from build123d import *

# Parameters (mm, degrees)
F0_W     = 10
F0_H     = 12
F0_W_2   = 7.6
F0_H_2   = 10
F1_DEPTH = 0.75
F0_W_3   = 6.8
F0_H_3   = 9.2
F2_DEPTH = 1.5
F3_R     = 1


with BuildPart() as f1:
    # F0 (on Top) → F1 (new body)
    with BuildSketch(Plane.XY):
        Rectangle(F0_W, F0_H)
        Rectangle(F0_W_2, F0_H_2, mode=Mode.SUBTRACT)
    extrude(amount=F1_DEPTH)

    # F0 (on Top) → F2 (join)
    with BuildSketch(Plane.XY):
        Rectangle(F0_W_2, F0_H_2)
        Rectangle(F0_W_3, F0_H_3, mode=Mode.SUBTRACT)
    extrude(amount=F2_DEPTH)

    # F3
    f3_edges = [f1.edges().sort_by_distance(p)[0] for p in [
        (5, 6, 0.375),
        (-5, 6, 0.375),
        (-5, -6, 0.375),
        (5, -6, 0.375),
    ]]
    fillet(f3_edges, radius=F3_R)


solid = f1.part
Work out the finished part from the listing and answer in its coordinate system (mm). A direction names the side the tool comes from. Give positions to 0.01 mm unless a question says otherwise; leave off trailing zeros. Order: outer loops, then holes, each group sorted by start corner. A loop starts at its lowest first (then second) coordinate and runs counter-clockwise, first axis right, second up. Notation, with made-up numbers: (-3.5, 79.5) -> (44.5, 79.5) arc R20 ccw to (44.5, 116.5) -> close; hole circle Ø11 at (-32, -3.5). An arc over 180 degrees is marked (long way). One line per item, written item: value.
Item 1: A tool of negligible diameter and unlimited length cuts with its end or side. For faces 1 (the cylindrical face through (-4.715, 5.699, 0.38)), 2 (the flat face through (0, 4.6, 1)), from which of +Z, -Z, +X, -X, +Y, -Y can it reach the whole face along a straight path? Write none if from no direction.
Answer sheet:
face 1: +Z, -Z, -X, +Y
face 2: +Z, -Z
Item 2: Find section C-C, the plane x = -1. Give the vertices of the cut face in (y, z).
Answer sheet:
outline: (-6, 0) -> (-4.6, 0) -> (-4.6, 1.5) -> (-5, 1.5) -> (-5, 0.75) -> (-6, 0.75) -> close; (4.6, 0) -> (6, 0) -> (6, 0.75) -> (5, 0.75) -> (5, 1.5) -> (4.6, 1.5) -> close
Item 3: Find section A-A, the plane y = -3.5. Give the vertices of the cut face in (x, z).
Answer sheet:
outline: (-5, 0) -> (-3.4, 0) -> (-3.4, 1.5) -> (-3.8, 1.5) -> (-3.8, 0.75) -> (-5, 0.75) -> close; (3.4, 0) -> (5, 0) -> (5, 0.75) -> (3.8, 0.75) -> (3.8, 1.5) -> (3.4, 1.5) -> close
Item 4: Determine the mould class of faces 3 (the flat face through (-4.5, 0.1, 0)), 4 (the cylindrical face through (4.699, -5.715, 0.38)), 5 (the cylindrical face through (4.699, 5.715, 0.38)), 6 (the flat face through (-3.4, 0, 1)) for opening direction Y: released by +Y, released by -Y, zero draft, split by the parting line, or undercut.
Answer sheet:
face 3: zero draft
face 4: released by -Y
face 5: released by +Y
face 6: undercut
Item 5: Find section D-D, the plane z = 1.05. Give the vertices of the cut face in (x, y), plus the area to 3 significant figures.
Answer sheet:
outline: (-3.8, -5) -> (3.8, -5) -> (3.8, 5) -> (-3.8, 5) -> close; hole (-3.4, -4.6) -> (3.4, -4.6) -> (3.4, 4.6) -> (-3.4, 4.6) -> close
area: 13.4 mm²
Item 6: Find section B-B, the plane z = 0.4. Give the vertices of the cut face in (x, y), plus the area to 3 significant figures.
Answer sheet:
outline: (-5, -5) arc R1 ccw to (-4, -6) -> (4, -6) arc R1 ccw to (5, -5) -> (5, 5) arc R1 ccw to (4, 6) -> (-4, 6) arc R1 ccw to (-5, 5) -> close; hole (-3.4, -4.6) -> (3.4, -4.6) -> (3.4, 4.6) -> (-3.4, 4.6) -> close
area: 56.6 mm²
Item 7: Straight lines are drawn through the part: probe 1 along X at (y, z) = (1.5, 0.9); probe 2 along Y at (x, z) = (1.5, 0.45); probe 3 along X at (y, z) = (0, 0.7). For each, find the intervals that lie inside material, in ascending order.
Answer sheet:
probe 1: -3.8 to -3.4, 3.4 to 3.8
probe 2: -6 to -4.6, 4.6 to 6
probe 3: -5 to -3.4, 3.4 to 5
